Geometry check sheet. Reference: drawing and pictorial views, mm from the part's lowest x, y, z. A direction names the side the tool comes from. Round coordinates to 2 decimals unless told otherwise and drop trailing zeros. Write each loop counter-clockwise with the first axis right and the second up, starting at its lowest first coordinate (ties: lowest second). Pieces come first, ordered by that corner, then holes. Notation, with made-up numbers: M 40,-37.75 L 82,-37.75 A27 cw 82,-10.75 Z; hole C -24.75,-26.75 d11. An arc over 180 degrees is marked long. One line per question, with ' | ' between items.
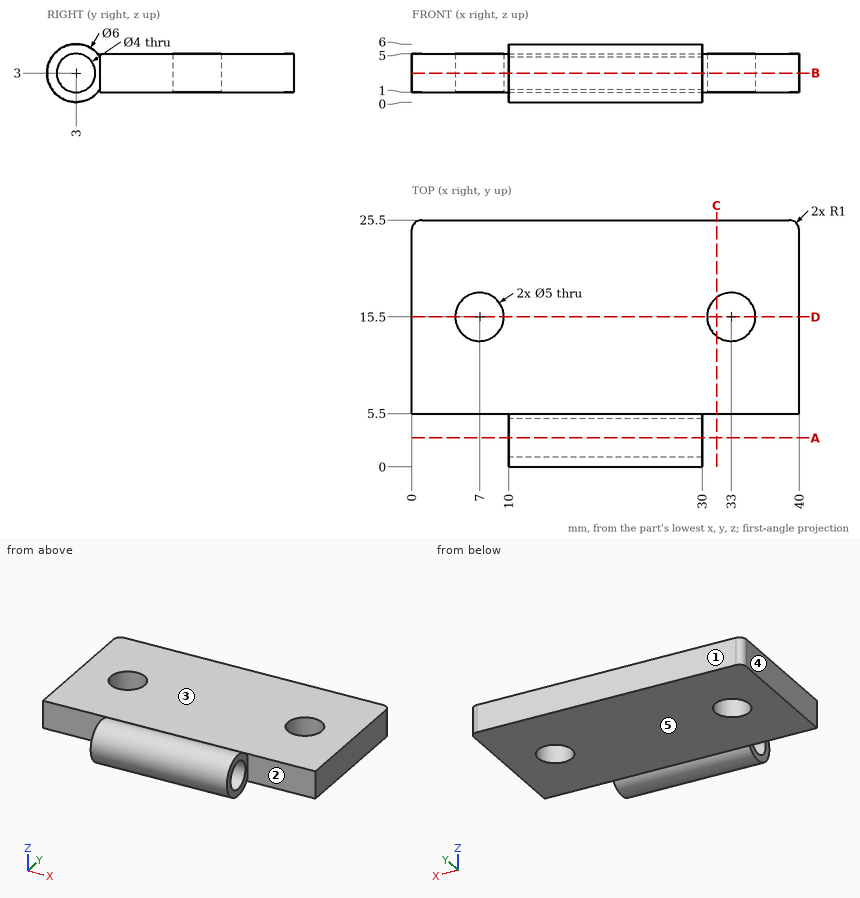
1. Tool access check on the marked faces 4 and 5. Record the directions out of +Z, -Z, +X, -X, +Y, -Y that give a thin tool (end or side, any length) a straight path to the whole face; none if there is none.
Results:
face 4: +Z, -Z, -X, +Y, -Y | face 5: -Z, +X, -X, +Y
2. Go/stop test with flat-tipped pins: P1, Ø3, axis at x = 20, y = 10, coming from the +Z side; P2, Ø5, axis at x = 10.5, y = 19.5, coming from the -Z side; P3, Ø3, axis at x = 15.5, z = 2, coming from the -Y side; P4, Ø1, axis at x = 11.5, z = 0.5, coming from the -Y side. Record where each tip stops, or that it passes through.
Results:
P1: stops at z = 5 | P2: stops at z = 1 | P3: stops at y = 0 | P4: stops at y = 0.76
3. Mould release check, pull along Y, two halves, no side actions. Record for the marked faces 1, 2 and 3: pulls with the +Y half, pulls with the -Y half, needs draft (parallel to the pull), parting line crosses it, or undercut.
Results:
face 1: pulls with the +Y half | face 2: undercut | face 3: needs draft
4. Section check C-C, the plane x = 31.5. Record the cut outline in (y, z).
Results:
outline: M 5.5,1 L 13.5,1 L 13.5,5 L 5.5,5 Z; M 17.5,1 L 25.5,1 L 25.5,5 L 17.5,5 Z
5. Thickness scan on line 1 (Y direction, x = 7, z = 3.25); line 2 (Y direction, x = 25, z = 3); line 3 (X direction, y = 17.5, z = 3.5). Record the ranges inside material, lowest first.
Results:
line 1: y = 5.5 to 13, 18 to 25.5 | line 2: y = 0 to 1, 5 to 25.5 | line 3: x = 0 to 5.5, 8.5 to 31.5, 34.5 to 40
6. Section check A-A, the plane y = 3. Record the cut outline in (x, z), then the cut area to 3 significant figures.
Results:
outline: M 10,0 L 30,0 L 30,1 L 10,1 Z; M 10,5 L 30,5 L 30,6 L 10,6 Z | area: 40.0 mm2
7. Section check B-B, the plane z = 3. Record the cut outline in (x, y), then the cut area to 3 significant figures.
Results:
outline: M 0,5.5 L 10,5.5 L 10,5 L 30,5 L 30,5.5 L 40,5.5 L 40,24.5 A1 ccw 39,25.5 L 1,25.5 A1 ccw 0,24.5 Z; M 10,0 L 30,0 L 30,1 L 10,1 Z; hole C 7,15.5 d5; hole C 33,15.5 d5 | area: 790 mm2
8. Section check D-D, the plane y = 15.5. Record the cut outline in (x, z).
Results:
outline: M 0,1 L 4.5,1 L 4.5,5 L 0,5 Z; M 9.5,1 L 30.5,1 L 30.5,5 L 9.5,5 Z; M 35.5,1 L 40,1 L 40,5 L 35.5,5 Z
